```python
from build123d import *

# Parameters (mm, degrees)
SKETCH1_R           = 4.75
BOSS_EXTRUDE1_DEPTH = 5
SKETCH2_R           = 4.5
CUT_EXTRUDE1_DEPTH  = 4


with BuildPart() as part:
    # Sketch1 → Boss-Extrude1 (new body)
    with BuildSketch(Plane(origin=(0, 0, 0), x_dir=(1, 0, 0), z_dir=(0, 1, 0))):
        with BuildLine():
            Line((5.649139951, 8), (10.28, 8))
            ThreePointArc((10.28, 8), (13.815533906, 6.535533906), (15.28, 3))
            Line((15.28, 3), (15.28, -3))
            ThreePointArc((15.28, -3), (13.815533906, -6.535533906), (10.28, -8))
            Line((10.28, -8), (5.649139951, -8))
            Line((5.649139951, -8), (-8.529960299, -6.75))
            ThreePointArc((-8.529960299, -6.75), (-13.302950922, -4.772978995), (-15.28, 0))
            ThreePointArc((-15.28, 0), (-13.302950922, 4.772978995), (-8.529960299, 6.75))
            Line((-8.529960299, 6.75), (5.649139951, 8))
        make_face()
        with Locations(Location((-8.529960299, 0, 0), (0, 0, 270))):
            Circle(SKETCH1_R, mode=Mode.SUBTRACT)
    extrude(amount=BOSS_EXTRUDE1_DEPTH)

    # Sketch2 → Cut-Extrude1 (cut)
    with BuildSketch(Plane(origin=(0, 5, 0), x_dir=(1, 0, 0), z_dir=(0, 1, 0))):
        with Locations(Location((6.280039701, 0, 0), (0, 0, 270))):
            Circle(SKETCH2_R)
    extrude(amount=-CUT_EXTRUDE1_DEPTH, mode=Mode.SUBTRACT)


solid = part.part
```
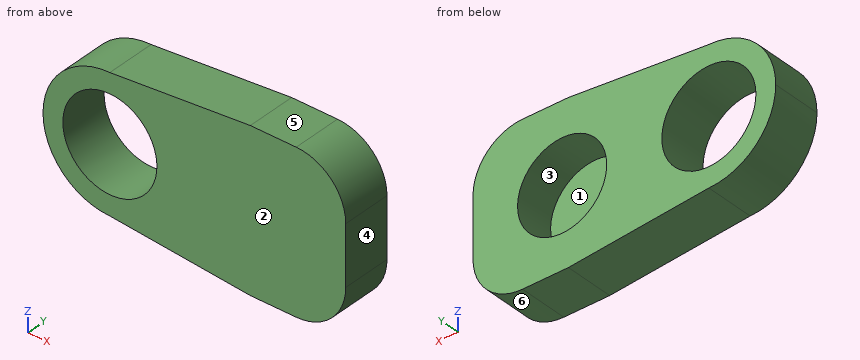
Can you work these out from the model? Positions are in its coordinate system, mm. Face numbers are marked on the shaded views. A direction names the side the tool comes from. Coordinates: 2 decimals unless noted, no trailing zeros. Loops run counter-clockwise (first coordinate to the right, second up) from the corner with the lowest first, then second, coordinate; pieces in that order, holes last. Notation, with made-up numbers: M 51.5,38 L 61.5,38 A29 ccw 61.5,68 Z; hole C 60.25,25 d4. An arc over 180 degrees is marked long. Put each result on its own line as item: value. Start each with the question number.
(1) Imagine slicing it at A-A on z = 2. List the corners of the cut face in (x, y) for me.
(2) Imagine slicing it at D-D on z = -4. List the corners of the cut face in (x, y) for me, and give its area (3 significant figures).
(3) Imagine slicing it at B-B on y = 4.35. List the corners of the cut face in (x, z) for me.
(4) We'd pull the mould along Z, two halves only. Please class the marked faces 3, 4, 5 and 6: +Z half, -Z half, draft (parallel to the pull), parting line (faces both ways), or undercut.
(5) I need wall thicknesses on probe 1 along X at (y, z) = (3.3, 0); probe 2 along Y at (x, z) = (7, -2); probe 3 along X at (y, z) = (1.7, 2.75). Which ranges of each line are inside material? Lowest first, please.
(6) Imagine slicing it at C-C on x = -7.5. List the corners of the cut face in (y, z) for me.
(7) Will these pins go through, and if not, where does the flat tip stop? pin 1 Ø2 at (x, y) = (1, 2.5) entering from +Z; pin 2 Ø4.5 at (x, z) = (7.5, -0.5) entering from +Y.
(8) Which directions (+Z, -Z, +X, -X, +Y, -Y) give clear straight access to the entire face, cutting with the end or side of a thin tool? Please do the marked faces 1 and 2.
Worked answers:
1. outline: M -14.98,0 L -12.84,0 L -12.84,5 L -14.98,5 Z; M -4.22,0 L 15.28,0 L 15.28,5 L 10.31,5 L 10.31,1 L 2.25,1 L 2.25,5 L -4.22,5 Z
2. outline: M -13.97,0 L -11.09,0 L -11.09,5 L -13.97,5 Z; M -5.97,0 L 15.18,0 L 15.18,5 L 8.34,5 L 8.34,1 L 4.22,1 L 4.22,5 L -5.97,5 Z
2. area: 104 mm2
3. outline: M -15.28,0 A6.75 ccw -8.53,-6.75 L 5.65,-8 L 10.28,-8 A5 ccw 15.28,-3 L 15.28,3 A5 ccw 10.28,8 L 5.65,8 L -8.53,6.75 A6.75 ccw Z; hole C -8.53,0 d9.5; hole C 6.28,0 d9
4. face 3: undercut
4. face 4: draft
4. face 5: +Z half
4. face 6: -Z half
5. probe 1: x = -15.28 to -13.28, -3.78 to 1.78, 10.78 to 15.28
5. probe 2: y = 0 to 1
5. probe 3: x = -14.69 to -12.4, -4.66 to 2.72, 9.84 to 15.28
6. outline: M 0,-6.84 L 5,-6.84 L 5,-4.64 L 0,-4.64 Z; M 0,4.64 L 5,4.64 L 5,6.84 L 0,6.84 Z
7. pin 1: stops at z = 7.68
7. pin 2: stops at y = 1
8. face 1: +Y
8. face 2: +Z, -Z, +X, -X, -Y
